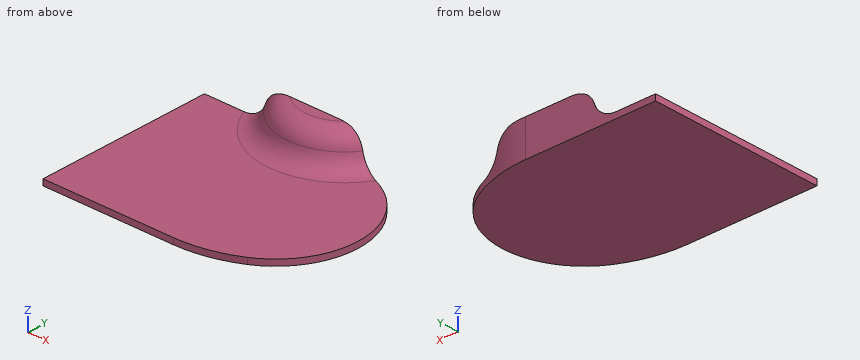
Autodesk Inventor part; units mm, degrees
ref_plane "YZ Plane" through (0, 0, 0) normal (1, 0, 0) x (0, 1, 0)
ref_plane "XZ Plane" through (0, 0, 0) normal (0, 1, 0) x (-1, 0, 0)
ref_plane "XY Plane" through (0, 0, 0) normal (0, 0, 1) x (1, 0, 0)
sketch "Sketch1" plane through (0, 0, 0) normal (0, 0, 1) x (1, 0, 0)
  line L0 (-4.4, 49.4) -> (30, 49.4)
  line L1 (-4.4, -37.6) -> (30, -37.6)
  line L2 (-4.4, -37.6) -> (90.6, -37.6)
  line L3 (90.6, -37.6) -> (90.6, 49.4)
  line L4 (90.6, 49.4) -> (-4.4, 49.4)
  line L5 (-4.4, 49.4) -> (-4.4, -37.6)
  point P0 (0, 0)
  dimension "d0" = 95
extrude "Extrusion1" add sketch "Sketch1" against normal blind 3
sketch "Sketch2" plane through (90.6, -37.6, 0) normal (1, 0, 0) x (0, 0, -1)
  circle A0 centre (17.5922, 43.5) radius 28.5 construction
  point P0 (0, 37.6)
  dimension "d5" = 57
sketch "Sketch3" plane through (0, 0, 0) normal (0, 0, 1) x (1, 0, 0)
  line L0 (90.6, 49.4) -> (-4.4, 49.4)
  line L1 (-4.4, 49.4) -> (-4.4, -37.6)
  line L2 (-4.4, -37.6) -> (90.6, -37.6)
  line L3 (90.6, -37.6) -> (90.6, 49.4)
  line L4 (90.6, 49.4) -> (-4.4, 49.4)
  line L5 (-4.4, 49.4) -> (90.6, 49.4)
  arc A0 (25.8108, 49.4) -> (78.1488, 49.4) centre (51.9798, 64.0691) ccw
  point P0 (0, 0)
  point P1 (25.8108, 49.4)
  point P2 (78.1488, 49.4)
  dimension "d9" = 30
extrude "Extrusion2" add sketch "Sketch3" along normal blind 15 contours A0 L0
sketch "Sketch4" plane through (-4.4, 49.4, -3) normal (0, 1, 0) x (1, 0, 0)
  point P0 (4.4, -3)
fillet "Fillet2" radius 10 2 edges at (51.9798, 34.0691, 15) (51.9798, 34.0691, 0)
sketch "Sketch7" plane through (0, 0, -3) normal (0, 0, -1) x (-1, 0, 0)
  line L0 (4.4, 49.4) -> (-90.6, 49.4)
  line L1 (-90.6, 49.4) -> (-90.6, -37.6)
  line L2 (-90.6, -37.6) -> (4.4, -37.6)
  line L3 (4.4, -37.6) -> (4.4, 49.4)
  line L4 (-90.6, -37.6) -> (4.4, -37.6)
  arc A0 (-90.6, -30.1) -> (-60.6, -37.6) centre (-60.6, 26.15) ccw
  line L5 (-90.6, 49.4) -> (-90.6, -37.6)
  line L6 (-90.6, 5.9) -> (-40.6, 5.9) construction
  arc A1 (-60.6, 49.4) -> (-90.6, 41.9) centre (-60.6, -14.35) ccw
  point P0 (0, 0)
  point P1 (-60.6, -37.6)
  dimension "d11" = 30
  dimension "d12" = 7.5
  dimension "d13" = 50
extrude "Extrusion3" cut sketch "Sketch7" against normal through all contours A1 L1 L0 | L2 L1 A0
sketch "Sketch8" plane through (0, 0, -3) normal (0, 0, -1) x (-1, 0, 0)
  arc A0 (-60.6, 49.4) -> (-90.6, 41.9) centre (-60.6, -14.35) ccw
  line L0 (-90.6, 41.9) -> (-90.6, -30.1)
  arc A1 (-90.6, -30.1) -> (-60.6, -37.6) centre (-60.6, 26.15) ccw
  line L1 (-60.6, -37.6) -> (4.4, -37.6)
  line L2 (4.4, -37.6) -> (4.4, 49.4)
  line L3 (4.4, 49.4) -> (-60.6, 49.4)
  arc A2 (-90.6, -30.1) -> (-60.6, -37.6) centre (-60.6, 26.15) ccw
  arc A3 (-90.6, 41.9) -> (-90.6, -30.1) centre (-71.4, 5.9) ccw
  point P0 (0, 0)
extrude "Extrusion4" add sketch "Sketch8" against normal blind 3 contours L0 A3
sketch "Sketch9" plane through (0, 0, -3) normal (0, 0, -1) x (-1, 0, 0)
  line L0 (-52.7475, -27.5099) -> (-72.7475, -27.5099)
  line L1 (-72.7475, -27.5099) -> (-72.7475, -34.5099)
  line L2 (-72.7475, -34.5099) -> (-52.7475, -34.5099)
  line L3 (-52.7475, -34.5099) -> (-52.7475, -27.5099)
  line L4 (4.4, -37.6) -> (4.4, 49.4)
  line L5 (4.4, 5.9) -> (-145.6, 5.9) construction
  line L6 (-52.7475, 39.3099) -> (-72.7475, 39.3099)
  line L7 (-72.7475, 39.3099) -> (-72.7475, 46.3099)
  line L8 (-72.7475, 46.3099) -> (-52.7475, 46.3099)
  line L9 (-52.7475, 46.3099) -> (-52.7475, 39.3099)
  point P0 (0, 0)
  dimension "d19" = 20
  dimension "d20" = 7
  dimension "d21" = 150
extrude "Extrusion5" [suppressed]
sketch "Sketch10" plane through (0, 0, 0) normal (0, 0, 1) x (1, 0, 0)
  line L0 (0.15, 35.15) -> (22.95, 35.15)
  line L1 (6.4671, 26.3395) -> (10.4671, 29.307)
  line L2 (-4.4, 32.9) -> (30, 32.9)
  arc A0 (90.6, 41.9) -> (85.9332, 44.1503) centre (60.6, -14.35) ccw
  line L3 (15.4501, 49.4) -> (-4.4, 49.4)
  line L4 (-4.4, 49.4) -> (-4.4, -37.6)
  line L5 (-4.4, -37.6) -> (60.6, -37.6)
  arc A1 (60.6, -37.6) -> (90.6, -30.1) centre (60.6, 26.15) ccw
  arc A2 (90.6, -30.1) -> (90.6, 41.9) centre (71.4, 5.9) ccw
  line L6 (-4.4, 49.4) -> (60.6, 49.4)
  arc A3 (3.8712, 49.4) -> (-4.4, 18.2775) centre (37.3788, 23.8346) ccw
  line L7 (60.6, -37.6) -> (-4.4, -37.6)
  arc A4 (-4.4, 18.2775) -> (19.2096, -37.6) centre (64.8355, 14.6046) ccw
  point P0 (0, 0)
sketch "Sketch12" plane through (-4.4, 49.4, 0) normal (0, 1, 0) x (1, 0, 0)
  line L0 (36.1854, -19.7901) -> (34.9706, -16.4151)
  line L1 (34.9706, -16.4151) -> (30.2063, -18.8238)
  line L2 (29.3711, -16.5035) -> (30.2063, -18.8238)
  line L3 (34.1354, -14.0948) -> (29.3711, -16.5035)
  line L4 (34.1354, -14.0948) -> (33.0724, -11.1417)
  line L5 (33.0724, -11.1417) -> (62.871, 3.9237)
  line L6 (67.8822, -9.9981) -> (62.871, 3.9237)
  line L7 (38.0836, -25.0635) -> (67.8822, -9.9981)
  line L8 (38.0836, -25.0635) -> (37.0206, -22.1104)
  line L9 (37.0206, -22.1104) -> (32.2563, -24.5191)
  line L10 (31.4211, -22.1988) -> (32.2563, -24.5191)
  line L11 (36.1854, -19.7901) -> (31.4211, -22.1988)
  line L12 (65, -15) -> (65, 3)
  line L13 (0, 3) -> (65, 3)
  line L14 (0, 0) -> (0, 3)
  line L15 (19.8501, 0) -> (0, 0)
  line L16 (65, -15) -> (42.785, -15)
  point P0 (4.4, 0)
properties part number "Palma"
Input: part model. Units: mm. Frame: model coordinates. Coordinates: 2 decimals unless noted, no trailing zeros. Write each loop counter-clockwise with the first axis right and the second up, starting at its lowest first coordinate (ties: lowest second). Pieces come first, ordered by that corner, then holes.
1) Section B-B on x = 5.5. Output: boundary loops of the cut face in (y, z).
2) Section C-C on y = -26. Output: boundary loops of the cut face in (x, z).
3) Material intervals for line 1 along Z through (x, y) = (76, -20); line 2 along Y through (x, z) = (98.5, -1.75); line 3 along X through (y, z) = (-10.5, -1), sorted ascending.
4) Section A-A on z = -1.25. Output: boundary loops of the cut face in (x, y).
5) Section D-D on z = 12.75. Output: boundary loops of the cut face in (x, y).
6) Pin query (flat end, axial travel): pin 1 Ø12 at (x, y) = (89, -14) entering from +Z; pin 2 Ø5 at (x, y) = (36, 38.5) entering from +Z; pin 3 Ø6 at (y, z) = (-18.5, 5) entering from +X; pin 4 Ø4 at (x, y) = (71, 29.5) entering from +Z. Return the tip coordinate at first contact, or that it passes through.
Check result:
1. outline: (-37.6, -3) - (49.4, -3) - (49.4, 0) - (-37.6, 0) - close
2. outline: (-4.4, -3) - (96.84, -3) - (96.84, 0) - (-4.4, 0) - close
3. line 1: z = -3 to 0
3. line 2: y = -24.6 to 36.4
3. line 3: x = -4.4 to 108.76
4. outline: (-4.4, -37.6) - (60.6, -37.6) arc R63.75 ccw to (90.6, -30.1) arc R40.8 ccw to (90.6, 41.9) arc R63.75 ccw to (60.6, 49.4) - (-4.4, 49.4) - close
5. outline: (30.13, 49.4) arc R26.32 ccw to (72.97, 48.19) arc R63.75 ccw to (60.6, 49.4) - close
6. pin 1: stops at z = 0
6. pin 2: stops at z = 11.44
6. pin 3: passes through
6. pin 4: stops at z = 0.18
